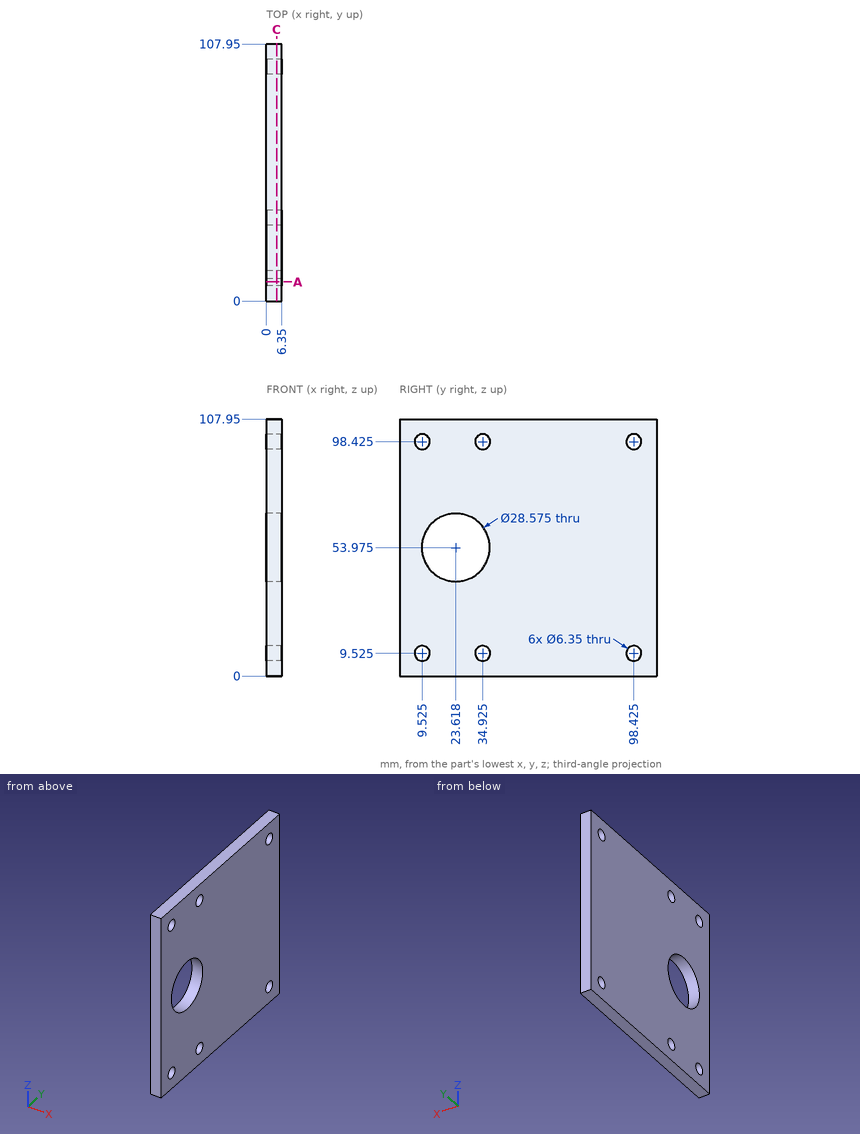
Study the drawing (mm; zero at the part's minimum x, y, z) and answer. Coordinates: 2 decimals unless noted, no trailing zeros. Order: outer loops, then holes, each group sorted by start corner. A loop starts at its lowest first (then second) coordinate and runs counter-clockwise, first axis right, second up. Notation, with made-up numbers: M -20.5,25.5 L 4.5,25.5 A22 ccw 4.5,61.5 Z; hole C -15.5,70.25 d2. An arc over 180 degrees is marked long. Use CSV: the item, a comma, the result in double quotes.
Q1. Straight lines are drawn through the part: L1, parallel to Z at x = 5.5, y = 98; L2, parallel to Z at x = 1.25, y = 99.5; L3, parallel to Y at x = 2.25, z = 99.5. For each, find the intervals that lie inside material, in ascending order.
Here are the results:
L1,"0 to 6.38, 12.67 to 95.28, 101.57 to 107.95"
L2,"0 to 6.54, 12.51 to 95.44, 101.41 to 107.95"
L3,"0 to 6.54, 12.51 to 31.94, 37.91 to 95.44, 101.41 to 107.95"
Q2. Section C-C (x = 4.25) is taken. Give the number of separate pieces and of enclosed holes in the cut face, then the cut area to 3 significant figures.
Here are the results:
separate pieces,"1"
enclosed holes,"7"
area,"10,800 mm2"
Q3. Given pin 1 Ø4 at (y, z) = (34.925, 98.425) entering from +X, flat-ended and moving along its own axis, determine where the tip first touches the part or whether it passes through.
Here are the results:
pin 1,"through"
Q4. Section A-A (y = 8) is taken. Determine the outline of the cut face in (x, z).
Here are the results:
outline,"M 0,0 L 6.35,0 L 6.35,6.74 L 0,6.74 Z; M 0,12.31 L 6.35,12.31 L 6.35,95.64 L 0,95.64 Z; M 0,101.21 L 6.35,101.21 L 6.35,107.95 L 0,107.95 Z"
